from build123d import *

# Parameters (mm, degrees)
BASPROSKE_W        = 10
BASPROSKE_H        = 8.5
TOOTHCUT_DEPTH     = 16.636495771
TEETHCUTS_COUNT    = 15
TEETHCUTS_ANGLE    = 336
BORSKE_R           = 0.4
BORE_DEPTH         = 50.0000508
CUT_EXTRUDE1_REACH = 17.622
SKETCH1_R          = 1.5


with BuildPart() as part:
    # BasProSke → Base-Revolve (revolve)
    with BuildSketch(Plane(origin=(0, 0, 0), x_dir=(1, 0, 0), z_dir=(0, 1, 0)), mode=Mode.PRIVATE) as base_revolve_sk:
        with Locations((5, 4.25)):
            Rectangle(BASPROSKE_W, BASPROSKE_H)
    revolve(base_revolve_sk.sketch.rotate(Axis((-10, 0, 0), (1, 0, 0)), 180), axis=Axis((-10, 0, 0), (1, 0, 0)))

    # TooCutSke → ToothCut (cut, through all)
    with BuildSketch(Plane(origin=(0, 0, 0), x_dir=(0, 0, -1), z_dir=(1, 0, 0))):
        with BuildLine():
            ThreePointArc((0.531576138, 6.226349477), (0, 6.249), (-0.531576138, 6.226349477))
            ThreePointArc((-0.531576138, 6.226349477), (-0.830301624, 7.411024729), (-1.576608494, 8.378350125))
            ThreePointArc((-1.576608494, 8.378350125), (0, 8.5254), (1.576608494, 8.378350125))
            ThreePointArc((1.576608494, 8.378350125), (0.830301624, 7.411024729), (0.531576138, 6.226349477))
        make_face()
    toothcut = extrude(amount=TOOTHCUT_DEPTH, mode=Mode.SUBTRACT)

    # TeethCuts: ToothCut ×15 about axis
    teethcuts_axis = Axis((-10, 0, 0), (1, 0, 0))
    for i in range(1, TEETHCUTS_COUNT):
        add(toothcut.rotate(teethcuts_axis, i * TEETHCUTS_ANGLE / (TEETHCUTS_COUNT - 1)), mode=Mode.SUBTRACT)

    # BorSke → Bore (cut, symmetric)
    with BuildSketch(Plane(origin=(0, 0, 0), x_dir=(0, 0, -1), z_dir=(1, 0, 0))):
        with Locations(Location((0, 0, 0), (0, 0, 180))):
            Circle(BORSKE_R)
    extrude(amount=BORE_DEPTH, both=True, mode=Mode.SUBTRACT)

    # Sketch1 → Cut-Extrude1 (cut, up to next)
    with BuildSketch(Plane(origin=(10, 0, 0), x_dir=(0, 0, -1), z_dir=(1, 0, 0)), mode=Mode.PRIVATE) as cut_extrude1_sk1:
        Circle(SKETCH1_R)
    cut_extrude1_tool1 = extrude(cut_extrude1_sk1.sketch, amount=-CUT_EXTRUDE1_REACH, mode=Mode.PRIVATE) & part.part
    add(cut_extrude1_tool1.solids().sort_by_distance((10, 0, 0))[0], mode=Mode.SUBTRACT)


solid = part.part
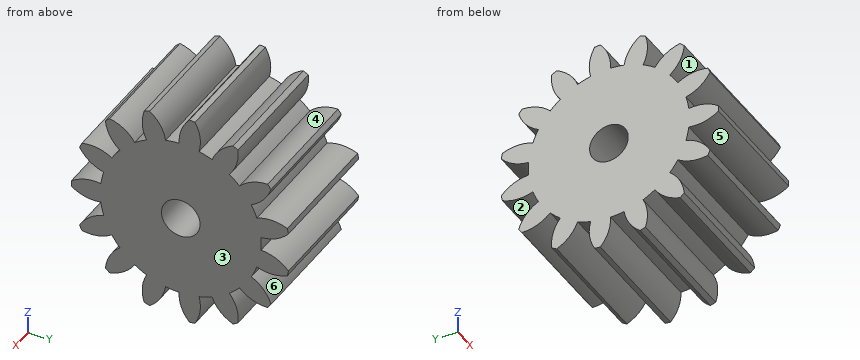
Design review of the part built by this model. Coordinates are the model's own, in mm. Face numbers are marked on the shaded views. A direction names the side the tool comes from. Give positions to 0.01 mm unless a question says otherwise; leave off trailing zeros. Order: outer loops, then holes, each group sorted by start corner. A loop starts at its lowest first (then second) coordinate and runs counter-clockwise, first axis right, second up. Notation, with made-up numbers: (2, -24.5) - (10, -24.5) arc R13 cw to (10, -13.5) - close; hole circle Ø10 at (67.25, -23). An arc over 180 degrees is marked (long way). Write item = value, one per line. Start each with the question number.
Q1. We need section A-A on z = 0. State the section outline as (x, y) points, plus the area to 3 significant figures.
Q2. Mouldability with a two-part tool opening along Y and no side actions: class the marked faces 1, 2 and 3 as released by +Y, released by -Y, zero draft, split by the parting line, or undercut.
Q3. We need section B-B on y = -4. State the section outline as (x, z) points, plus the area to 3 significant figures.
Q4. Clearance check with flat-ended pins moving along their axes: pin 1 Ø3.5 at (y, z) = (0, 0) entering from +X; pin 2 Ø3 at (x, y) = (1.5, -1) entering from -Z; pin 3 Ø6 at (x, y) = (1.5, 6) entering from -Z. State where each tip first meets the part, or that it passes through.
Q5. We need section C-C on y = 1.75. State the section outline as (x, z) points.
Q6. Tool access review of the marked faces 4, 5 and 6: name each direction out of +Z, -Z, +X, -X, +Y, -Y from which nothing blocks a thin tool from reaching the whole face with its end or side.
Q7. To check wall thickness, follow L1, parallel to Y at x = 5, z = 0; L2, parallel to Z at x = 3, y = -5.5; L3, parallel to Y at x = 4.5, z = -1.25. State the ranges of each line that lie inside material, in increasing order. Write a range as from..to.
Working result:
q1.outline = (0, -8.5) - (10, -8.5) - (10, -1.5) - (0, -1.5) - close; (0, 1.5) - (10, 1.5) - (10, 6.25) - (0, 6.25) - close
q1.area = 117 mm²
q2.face_1 = released by -Y
q2.face_2 = undercut
q2.face_3 = zero draft
q3.outline = (0, -5.65) - (10, -5.65) - (10, 5.65) - (0, 5.65) - close
q3.area = 113 mm²
q4.pin_1 = 10
q4.pin_2 = -8.27
q4.pin_3 = -7.47
q5.outline = (0, -6) - (10, -6) - (10, 6) - (0, 6) - close
q6.face_4 = +Z, +X, -X
q6.face_5 = +X, -X
q6.face_6 = +X, -X, +Y
q7.L1 = -8.5..-1.5, 1.5..6.25
q7.L2 = -6.46..-5.01, -3.32..3.32, 5.01..6.46
q7.L3 = -6.12..-0.83, 0.83..8.05
